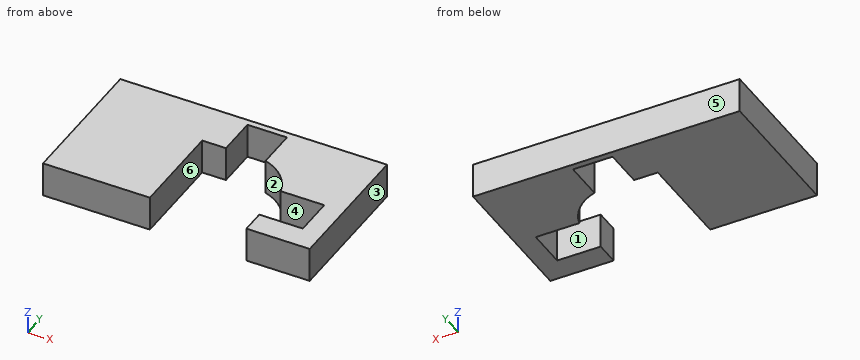
from build123d import *

# Parameters (mm, degrees)
BOSS_EXTRUDE1_DEPTH = 44


with BuildPart() as part:
    # Sketch2 → Boss-Extrude1 (new body)
    with BuildSketch(Plane.XY):
        with BuildLine():
            Line((-62.51623719, 80.614043502), (-32.51623719, 80.614043502))
            Line((-32.51623719, 80.614043502), (-32.51623719, 130.614043502))
            Line((-32.51623719, 130.614043502), (17.48376281, 130.614043502))
            Line((17.48376281, 130.614043502), (17.48376281, 80.614043502))
            ThreePointArc((17.48376281, 80.614043502), (43.840620434, 64.970901126), (59.48376281, 38.614043502))
            Line((59.48376281, 38.614043502), (114.48376281, 38.614043502))
            Line((114.48376281, 38.614043502), (114.48376281, -11.385956498))
            Line((114.48376281, -11.385956498), (59.48376281, -11.385956498))
            Line((59.48376281, -11.385956498), (59.48376281, -41.385956498))
            Line((59.48376281, -41.385956498), (139.48376281, -41.385956498))
            Line((139.48376281, -41.385956498), (139.48376281, 138.614043502))
            Line((139.48376281, 138.614043502), (-197.51623719, 138.614043502))
            Line((-197.51623719, 138.614043502), (-197.51623719, -41.385956498))
            Line((-197.51623719, -41.385956498), (-62.51623719, -41.385956498))
            Line((-62.51623719, -41.385956498), (-62.51623719, 80.614043502))
        make_face()
    extrude(amount=BOSS_EXTRUDE1_DEPTH)


solid = part.part
Can you work these out from the model? Positions are in its coordinate system, mm. Face numbers are marked on the shaded views. A direction names the side the tool comes from. Round coordinates to 2 decimals unless told otherwise and drop trailing zeros. Order: outer loops, then holes, each group sorted by start corner. A loop starts at its lowest first (then second) coordinate and runs counter-clockwise, first axis right, second up. Notation, with made-up numbers: M 22,75.25 L 34,75.25 A14 ccw 34,86.25 Z; hole C 46,59.5 d9. An arc over 180 degrees is marked long. Use a Markdown table: item, result.
1) Imagine slicing it at D-D (x = -21.5). List the corners of the cut face in (y, z) for me, then the cut area to 3 significant figures.
Geometry says:
| item | result |
|---|---|
| outline | M 130.61,0 L 138.61,0 L 138.61,44 L 130.61,44 Z |
| area | 352 mm² |
2) Imagine slicing it at A-A (y = 103). List the corners of the cut face in (x, z) for me, then the cut area to 3 significant figures.
Geometry says:
| item | result |
|---|---|
| outline | M -197.52,0 L -32.52,0 L -32.52,44 L -197.52,44 Z; M 17.48,0 L 139.48,0 L 139.48,44 L 17.48,44 Z |
| area | 12,600 mm² |
3) On a 3-axis mill with a long thin cutter (end or side, diameter ignored), from which of +Z, -Z, +X, -X, +Y, -Y can I reach the whole of each face in a straight line? I mean the marked faces 4, 5 and 6. Say none if no direction works.
Geometry says:
| item | result |
|---|---|
| face 4 | +Z, -Z |
| face 5 | +Z, -Z, +X, -X, +Y |
| face 6 | +Z, -Z, -Y |
4) If I drill on line 1 along X through (y, z) = (18, 29); line 2 along Y through (x, z) = (78.5, 41); line 3 along X through (y, z) = (99, 22), over which ranges is the centre line in solid material (lowest first)?
Geometry says:
| item | result |
|---|---|
| line 1 | x = -197.52 to -62.52, 114.48 to 139.48 |
| line 2 | y = -41.39 to -11.39, 38.61 to 138.61 |
| line 3 | x = -197.52 to -32.52, 17.48 to 139.48 |
5) I'm going to push flat-ended pins straight in: P1, Ø9, axis at x = -45, z = 31.5, coming from the -Y side; P2, Ø1.5, axis at x = -26, z = 19, coming from the -Y side. Where does each tip first touch, or does it pass through?
Geometry says:
| item | result |
|---|---|
| P1 | stops at y = 80.61 |
| P2 | stops at y = 130.61 |
6) Imagine slicing it at C-C (y = -29.5). List the corners of the cut face in (x, z) for me, then the cut area to 3 significant figures.
Geometry says:
| item | result |
|---|---|
| outline | M -197.52,0 L -62.52,0 L -62.52,44 L -197.52,44 Z; M 59.48,0 L 139.48,0 L 139.48,44 L 59.48,44 Z |
| area | 9,460 mm² |
7) If we mould it in two halves opening along Y, with no side actions, what happens to the marked faces 1, 2 and 3? For each: +Y half, -Y half, draft (parallel to the pull), parting line (faces both ways), or undercut.
Geometry says:
| item | result |
|---|---|
| face 1 | undercut |
| face 2 | -Y half |
| face 3 | draft |
8) Imagine slicing it at B-B (z = 8.5). List the corners of the cut face in (x, y) for me.
Geometry says:
| item | result |
|---|---|
| outline | M -197.52,-41.39 L -62.52,-41.39 L -62.52,80.61 L -32.52,80.61 L -32.52,130.61 L 17.48,130.61 L 17.48,80.61 A62 cw 59.48,38.61 L 114.48,38.61 L 114.48,-11.39 L 59.48,-11.39 L 59.48,-41.39 L 139.48,-41.39 L 139.48,138.61 L -197.52,138.61 Z |
